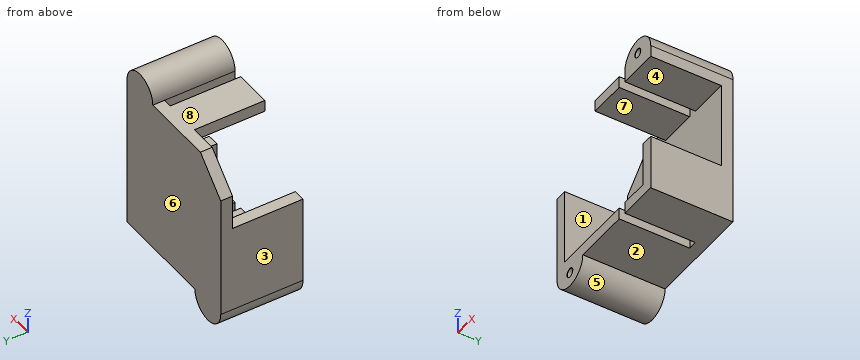
```python
from build123d import *

# Parameters (mm, degrees)
SKETCH_1_W             = 15.44
SKETCH_1_H             = 16.82
EXTRUDE_1_DEPTH        = 9
SHELL_3_T              = 1.5
SKETCH_2_W             = 1.5
SKETCH_2_H             = 11.15
CUT_EXTRUDE_1_DEPTH    = 9
SKETCH_3_W             = 7.5
SKETCH_3_H             = 8.5
CUT_EXTRUDE_2_DEPTH    = 9
SKETCH_4_W             = 1.12
SKETCH_4_H             = 1.5
CUT_EXTRUDE_3_DEPTH    = 9
CHAMFER_1_SIZE         = 4
EXTRUDE_2_REACH        = 19.131
M1_4X0_3_1_D           = 1.1
M1_4X0_3_1_DEPTH       = 7.66952666
M1_4X0_3_1_CSINK_D     = 1.15
M1_4X0_3_1_CSINK_ANGLE = 90
M1_4X0_3_1_TIP         = 0.33047334


with BuildPart() as part:
    # 草图1 → 凸台-拉伸1 (new body)
    with BuildSketch(Plane(origin=(0, 0, 0), x_dir=(1, 0, 0), z_dir=(0, 1, 0))):
        Rectangle(SKETCH_1_W, SKETCH_1_H)
    extrude(amount=EXTRUDE_1_DEPTH)

    # 抽壳3
    shell_3_openings = [part.faces().sort_by_distance(p)[0] for p in [
        (0, 0, 0),
    ]]
    offset(amount=SHELL_3_T, openings=shell_3_openings, kind=Kind.INTERSECTION)

    # 草图2 → 切除-拉伸1 (cut)
    with BuildSketch(Plane.XZ):
        with Locations((8.47, 2.835)):
            Rectangle(SKETCH_2_W, SKETCH_2_H)
    extrude(amount=-CUT_EXTRUDE_1_DEPTH, mode=Mode.SUBTRACT)

    # 草图3 → 切除-拉伸2 (cut)
    with BuildSketch(Plane.XZ):
        with Locations((-5.47, 5.66)):
            Rectangle(SKETCH_3_W, SKETCH_3_H)
    extrude(amount=-CUT_EXTRUDE_2_DEPTH, mode=Mode.SUBTRACT)

    # 草图4 → 切除-拉伸3 (cut)
    with BuildSketch(Plane.XZ):
        with Locations((3.58, 9.16)):
            Rectangle(SKETCH_4_W, SKETCH_4_H)
        with Locations((3.58, -9.16)):
            Rectangle(SKETCH_4_W, SKETCH_4_H)
    extrude(amount=-CUT_EXTRUDE_3_DEPTH, mode=Mode.SUBTRACT)

    # 倒角1
    chamfer_1_edges = [part.edges().sort_by_distance(p)[0] for p in [
        (-9.22, 9.75, 9.91),
    ]]
    chamfer(chamfer_1_edges, length=CHAMFER_1_SIZE)

    # 凸台-拉伸2: up to this face of the body (flat: up to its plane)
    extrude_2_end = Plane(part.part.faces().sort_by_distance((0.176494327, 10.5, -0.191935716))[0])
    # 草图5 → 凸台-拉伸2 (add, up to the picked face)
    with BuildSketch(Plane.XZ, mode=Mode.PRIVATE) as extrude_2_sk1:
        with BuildLine():
            Line((9.22, 9.91), (4.14, 9.91))
            ThreePointArc((4.14, 9.91), (6.68, 12.45), (9.22, 9.91))
        make_face()
    extrude_2_tool1 = split(extrude(extrude_2_sk1.sketch, amount=-EXTRUDE_2_REACH, mode=Mode.PRIVATE), bisect_by=extrude_2_end, keep=Keep.BOTH, mode=Mode.PRIVATE)
    # 草图5 → 凸台-拉伸2 (add, up to the picked face)
    with BuildSketch(Plane.XZ, mode=Mode.PRIVATE) as extrude_2_sk2:
        with BuildLine():
            Line((-9.22, -9.91), (-4.14, -9.91))
            ThreePointArc((-4.14, -9.91), (-6.68, -12.45), (-9.22, -9.91))
        make_face()
    extrude_2_tool2 = split(extrude(extrude_2_sk2.sketch, amount=-EXTRUDE_2_REACH, mode=Mode.PRIVATE), bisect_by=extrude_2_end, keep=Keep.BOTH, mode=Mode.PRIVATE)
    add(extrude_2_tool1.solids().sort_by(Axis((6.68, 0, 10.988009), (0, 1, 0)))[0])
    add(extrude_2_tool2.solids().sort_by(Axis((-6.68, 0, -10.988009), (0, 1, 0)))[0])

    # M1.4X0.3 螺纹孔的螺纹孔钻头1
    with Locations(Plane(origin=(0, 0, 0), x_dir=(-1, 0, 0), z_dir=(0, -1, 0))):
        with Locations((6.68, 10.63), (-6.68, -10.63)):
            CounterSinkHole(M1_4X0_3_1_D / 2, M1_4X0_3_1_CSINK_D / 2, depth=M1_4X0_3_1_DEPTH, counter_sink_angle=M1_4X0_3_1_CSINK_ANGLE)
            with Locations((0, 0, -(M1_4X0_3_1_DEPTH + M1_4X0_3_1_TIP / 2))):  # 118° drill point
                Cone(0, M1_4X0_3_1_D / 2, M1_4X0_3_1_TIP, mode=Mode.SUBTRACT)


solid = part.part
```
Verification items for the finished model (mm, model axes). Face numbers are marked on the shaded views. A direction names the side the tool comes from. Give positions to 0.01 mm unless a question says otherwise; leave off trailing zeros. Order: outer loops, then holes, each group sorted by start corner. A loop starts at its lowest first (then second) coordinate and runs counter-clockwise, first axis right, second up. Notation, with made-up numbers: (-13.75, 19) -> (18.25, 19) arc R27 cw to (18.25, 53) -> close; hole circle Ø4 at (-4, 9.25). An arc over 180 degrees is marked (long way). Use a Markdown table: item, result.
1) Section check D-D, the plane x = -3.5. Record the boundary of the cut face in (y, z), then the cut area to 3 significant figures.
Results:
| item | result |
|---|---|
| outline | (0, -9.91) -> (10.5, -9.91) -> (10.5, 9.91) -> (9, 9.91) -> (9, -8.41) -> (0, -8.41) -> close |
| area | 43.2 mm² |
2) Mould release check, pull along Z, two halves, no side actions. Record for the marked faces 5, 6, 7 and 8: pulls with the +Z half, pulls with the -Z half, needs draft (parallel to the pull), parting line crosses it, or undercut.
Results:
| item | result |
|---|---|
| face 5 | pulls with the -Z half |
| face 6 | needs draft |
| face 7 | undercut |
| face 8 | pulls with the +Z half |
3) Section check A-A, the plane y = 5.75. Record the boundary of the cut face in (x, z), then the cut area to 3 significant figures.
Results:
| item | result |
|---|---|
| outline | (-9.22, -9.91) arc R2.54 ccw to (-4.14, -9.91) -> (3.02, -9.91) -> (3.02, -8.41) -> (-7.72, -8.41) -> (-7.72, 1.41) -> (-9.22, 1.41) -> close; (-1.72, 8.41) -> (3.02, 8.41) -> (3.02, 9.91) -> (-1.72, 9.91) -> close; (4.14, -9.91) -> (9.22, -9.91) -> (9.22, -2.74) -> (7.72, -2.74) -> (7.72, -8.41) -> (4.14, -8.41) -> close; (4.14, 8.41) -> (9.22, 8.41) -> (9.22, 9.91) arc R2.54 ccw to (4.14, 9.91) -> close; hole circle Ø1.1 at (-6.68, -10.63); hole circle Ø1.1 at (6.68, 10.63) |
| area | 82.3 mm² |
4) Tool access check on the marked faces 1, 2, 3 and 4. Record the directions out of +Z, -Z, +X, -X, +Y, -Y that give a thin tool (end or side, any length) a straight path to the whole face; none if there is none.
Results:
| item | result |
|---|---|
| face 1 | +Z, -Y |
| face 2 | -Z, +X, +Y, -Y |
| face 3 | +Z, -Z, -X, +Y, -Y |
| face 4 | +X, -X, -Y |
5) Section check B-B, the plane z = -2. Record the boundary of the cut face in (x, y), then the cut area to 3 significant figures.
Results:
| item | result |
|---|---|
| outline | (-9.22, 0) -> (-7.72, 0) -> (-7.72, 9) -> (9.22, 9) -> (9.22, 10.5) -> (-9.22, 10.5) -> close |
| area | 41.2 mm² |
6) Section check C-C, the plane x = -0.5. Record the boundary of the cut face in (y, z), then the cut area to 3 significant figures.
Results:
| item | result |
|---|---|
| outline | (0, -9.91) -> (10.5, -9.91) -> (10.5, 9.91) -> (0, 9.91) -> (0, 8.41) -> (9, 8.41) -> (9, -8.41) -> (0, -8.41) -> close |
| area | 56.7 mm² |
7) Material ranges on probe 1 along Z at (x, y) = (6.68, 5); probe 2 along X at (y, z) = (7.5, -7.5); probe 3 along Z at (x, y) = (-6.68, 2.25), recorded low to high.
Results:
| item | result |
|---|---|
| probe 1 | -9.91 to -8.41, 8.41 to 10.08, 11.18 to 12.45 |
| probe 2 | -9.22 to -7.72, 7.72 to 9.22 |
| probe 3 | -12.45 to -11.18, -10.08 to -8.41 |
8) Depth check by flat-ended pin: pin 1 Ø5 at (x, y) = (-6.5, 8.5) entering from +Z; pin 2 Ø1.6 at (y, z) = (2.5, 9) entering from -X; pin 3 Ø1.5 at (x, y) = (-5, 7) entering from +Z. Enter the tip coordinate at first touch or a pass-through.
Results:
| item | result |
|---|---|
| pin 1 | z = 9.91 |
| pin 2 | x = -1.72 |
| pin 3 | z = -8.41 |
